from build123d import *

# Parameters (mm, degrees)
SKETCH2_R           = 50
BOSS_EXTRUDE1_DEPTH = 200
SKETCH4_W           = 314.300936027
SKETCH4_H           = 120
BOSS_EXTRUDE2_DEPTH = 200
SKETCH7_R           = 45
CUT_EXTRUDE1_DEPTH  = 121


with BuildPart() as part:
    # Sketch2 → Boss-Extrude1 (new body)
    with BuildSketch(Plane.XY):
        with BuildLine():
            Line((-32.872426913, -50.193660445), (-367.496829879, 168.955852308))
            ThreePointArc((-367.496829879, 168.955852308), (-384.818063411, 252.021939666), (-301.751976053, 269.343173198))
            Line((-301.751976053, 269.343173198), (32.872426913, 50.193660445))
            ThreePointArc((32.872426913, 50.193660445), (50.193660445, -32.872426913), (-32.872426913, -50.193660445))
        make_face()
        with Locations((-334.624402966, 219.149512753)):
            Circle(SKETCH2_R, mode=Mode.SUBTRACT)
    extrude(amount=BOSS_EXTRUDE1_DEPTH)

    # Sketch4 → Boss-Extrude2 (add)
    with BuildSketch(Plane.XY.offset(200)):
        with Locations((142.849531987, 0)):
            Rectangle(SKETCH4_W, SKETCH4_H)
    extrude(amount=-BOSS_EXTRUDE2_DEPTH)

    # Sketch7 → Cut-Extrude1 (cut, through all)
    with BuildSketch(Plane(origin=(0, 60, 0), x_dir=(1, 0, 0), z_dir=(0, 1, 0))):
        with Locations((163.399277188, -100)):
            Circle(SKETCH7_R)
    extrude(amount=-CUT_EXTRUDE1_DEPTH, mode=Mode.SUBTRACT)


solid = part.part
Work out the finished part from the listing and answer in its coordinate system (mm). Coordinates: 2 decimals unless noted, no trailing zeros. Write each loop counter-clockwise with the first axis right and the second up, starting at its lowest first coordinate (ties: lowest second). Pieces come first, ordered by that corner, then holes. Notation, with made-up numbers: (10.5, 36) - (35.5, 36) arc R6 cw to (35.5, 47) - close; hole circle Ø5 at (-16.5, -5.5). An arc over 180 degrees is marked (long way). One line per question, with ' | ' between items.
1) Consider probe 1 along Y at (x, z) = (259, 38.5); probe 2 along X at (y, z) = (24, 100); probe 3 along X at (y, z) = (-14.5, 125). Determine where each line is inside the solid, lowest interval first. Write a range as [from, to].
Checks:
probe 1: [-60, 60] | probe 2: [-146.16, 118.4], [208.4, 300] | probe 3: [-87.37, 125.98], [200.82, 300]
2) The mould has two halves that part along X. Classify faces 1 (the face through (-384.576, 221.348, 98.6)), 2 (the face through (157, 60, 146)), 3 (the face through (-23.799, -55.078, 98.6)): +X half, -X half, draft (parallel to the pull), parting line (faces both ways), or undercut.
Checks:
face 1: undercut | face 2: draft | face 3: -X half
3) Find section B-B, the plane y = 179.5. Determine the outline of the cut face in (x, z).
Checks:
outline: (-379.66, 0) - (-365.09, 0) - (-365.09, 200) - (-379.66, 200) - close; (-304.16, 0) - (-164.57, 0) - (-164.57, 200) - (-304.16, 200) - close
4) Find section A-A, the plane z = 130.5. Determine the outline of the cut face in (x, y), and give its area (3 significant figures).
Checks:
outline: (-367.5, 168.96) - (-32.87, -50.19) arc R60 ccw to (-14.3, -58.27) - (-14.3, -60) - (130.31, -60) - (130.31, 60) - (17.9, 60) - (-301.75, 269.34) arc R60 ccw to start; (196.49, -60) - (300, -60) - (300, 60) - (196.49, 60) - close; hole circle Ø100 at (-334.62, 219.15) | area: 73,800 mm2
5) Find section C-C, the plane z = 82. Determine the outline of the cut face in (x, y), and give its area (3 significant figures).
Checks:
outline: (-367.5, 168.96) - (-32.87, -50.19) arc R60 ccw to (-14.3, -58.27) - (-14.3, -60) - (122.16, -60) - (122.16, 60) - (17.9, 60) - (-301.75, 269.34) arc R60 ccw to start; (204.64, -60) - (300, -60) - (300, 60) - (204.64, 60) - close; hole circle Ø100 at (-334.62, 219.15) | area: 71,900 mm2
6) Flat-ended cylindrical pins translate along their axes: P1, Ø5, axis at y = 239.5, z = 133, coming from the +X side; P2, Ø10, axis at x = 116.5, z = 21, coming from the +Y side; P3, Ø1, axis at x = -218.5, z = 56.5, coming from the -Y side. Find the tip coordinate at first contact, or state that the pin passes through.
Checks:
P1: x = -252.37 | P2: y = 60 | P3: y = 71.05
7) Find section D-D, the plane x = 110.5. Determine the outline of the cut face in (y, z), and give its area (3 significant figures).
Checks:
outline: (-60, 0) - (60, 0) - (60, 200) - (-60, 200) - close | area: 24,000 mm2
